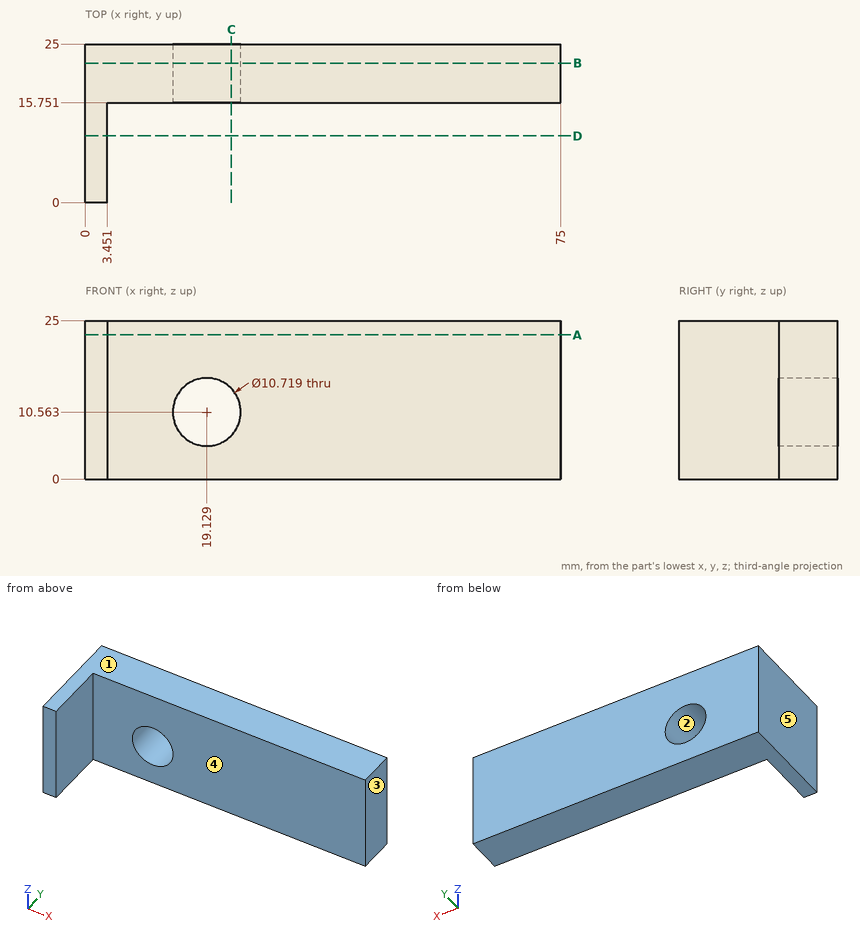
For this review, use the dimensioned drawing (mm, ordinates from the lowest corner) and the shaded views. A direction names the side the tool comes from. Give positions to 0.01 mm unless a question says otherwise; leave off trailing zeros. Order: outer loops, then holes, each group sorted by start corner. A loop starts at its lowest first (then second) coordinate and runs counter-clockwise, first axis right, second up. Notation, with made-up numbers: (83.25, -23.5) - (87.25, -23.5) arc R18 cw to (87.25, 7.5) - close; hole circle Ø7 at (81.5, -28). An arc over 180 degrees is marked (long way). Write item = value, one per line. Start each with the question number.
Q1. Mouldability with a two-part tool opening along Z and no side actions: class the marked faces 1, 2 and 3 as released by +Z, released by -Z, zero draft, split by the parting line, or undercut.
Q2. We need section B-B on y = 22. State the section outline as (x, z) points.
Q3. We need section D-D on y = 10.5. State the section outline as (x, z) points.
Q4. We need section C-C on x = 23. State the section outline as (y, z) points, plus the area to 3 significant figures.
Q5. Tool access review of the marked faces 4 and 5: name each direction out of +Z, -Z, +X, -X, +Y, -Y from which nothing blocks a thin tool from reaching the whole face with its end or side.
Q6. Clearance check with flat-ended pins moving along their axes: pin 1 Ø2 at (y, z) = (6.5, 3) entering from +X; pin 2 Ø14 at (x, z) = (19.13, 10.56) entering from -Y. State where each tip first meets the part, or that it passes through.
Q7. To check wall thickness, follow L1, parallel to X at y = 8, z = 19.75; L2, parallel to Y at x = 41.5, z = 20.25; L3, parallel to X at y = 23, z = 14 (1 decimal). State the ranges of each line that lie inside material, in increasing order. Write a range as from..to.
Q8. We need section A-A on z = 22.75. State the section outline as (x, y) points.
Working result:
q1.face_1 = released by +Z
q1.face_2 = undercut
q1.face_3 = zero draft
q2.outline = (0, 0) - (75, 0) - (75, 25) - (0, 25) - close; hole circle Ø10.72 at (19.13, 10.56)
q3.outline = (0, 0) - (3.45, 0) - (3.45, 25) - (0, 25) - close
q4.outline = (15.75, 0) - (25, 0) - (25, 6.86) - (15.75, 6.86) - close; (15.75, 14.27) - (25, 14.27) - (25, 25) - (15.75, 25) - close
q4.area = 163 mm²
q5.face_4 = +Z, -Z, +X, -Y
q5.face_5 = +Z, -Z, -X, +Y, -Y
q6.pin_1 = 3.45
q6.pin_2 = 15.75
q7.L1 = 0..3.45
q7.L2 = 15.75..25
q7.L3 = 0..15, 23.2..75
q8.outline = (0, 0) - (3.45, 0) - (3.45, 15.75) - (75, 15.75) - (75, 25) - (0, 25) - close
